from build123d import *

# Parameters (mm, degrees)
SKETCH2_W           = 17
SKETCH2_H           = 21
BOSS_EXTRUDE1_DEPTH = 3
SKETCH4_R           = 1.25
CUT_EXTRUDE1_DEPTH  = 6
SKETCH5_R           = 1.25
CUT_EXTRUDE2_DEPTH  = 6
SKETCH6_W           = 12
SKETCH6_H           = 10
BOSS_EXTRUDE3_DEPTH = 8
SKETCH7_W           = 5
SKETCH7_H           = 4
BOSS_EXTRUDE4_DEPTH = 4
BOSS_EXTRUDE5_DEPTH = 4
SKETCH9_R           = 1
CUT_EXTRUDE3_DEPTH  = 6


with BuildPart() as part:
    # Sketch2 → Boss-Extrude1 (new body)
    with BuildSketch(Plane(origin=(0, 0, 0), x_dir=(1, 0, 0), z_dir=(0, 1, 0))):
        with Locations((8.5, 10.5)):
            Rectangle(SKETCH2_W, SKETCH2_H)
    extrude(amount=BOSS_EXTRUDE1_DEPTH)

    # Sketch4 → Cut-Extrude1 (cut)
    with BuildSketch(Plane(origin=(0, 3, 0), x_dir=(1, 0, 0), z_dir=(0, 1, 0))):
        with Locations(Location((8, 18, 0), (0, 0, 270))):
            Circle(SKETCH4_R)
    extrude(amount=-CUT_EXTRUDE1_DEPTH, mode=Mode.SUBTRACT)

    # Sketch5 → Cut-Extrude2 (cut)
    with BuildSketch(Plane(origin=(0, 3, 0), x_dir=(1, 0, 0), z_dir=(0, 1, 0))):
        with Locations(Location((8, 3, 0), (0, 0, 270))):
            Circle(SKETCH5_R)
    extrude(amount=-CUT_EXTRUDE2_DEPTH, mode=Mode.SUBTRACT)

    # Sketch6 → Boss-Extrude3 (add)
    with BuildSketch(Plane(origin=(0, 3, 0), x_dir=(1, 0, 0), z_dir=(0, 1, 0))):
        with Locations((6, 10.5)):
            Rectangle(SKETCH6_W, SKETCH6_H)
    extrude(amount=BOSS_EXTRUDE3_DEPTH)

    # Sketch7 → Boss-Extrude4 (add)
    with BuildSketch(Plane(origin=(0, 3, 0), x_dir=(1, 0, 0), z_dir=(0, 1, 0))):
        with Locations((14.5, 10.5)):
            Rectangle(SKETCH7_W, SKETCH7_H)
    extrude(amount=BOSS_EXTRUDE4_DEPTH)

    # Sketch8 → Boss-Extrude5 (add)
    with BuildSketch(Plane(origin=(0, 0, -12.5), x_dir=(-1, 0, 0), z_dir=(0, 0, -1))):
        with BuildLine():
            Line((-17, 7), (-12, 7))
            Line((-12, 7), (-12, 11))
            ThreePointArc((-12, 11), (-15.234221224, 9.91777653), (-17, 7))
        make_face()
    extrude(amount=-BOSS_EXTRUDE5_DEPTH)

    # Sketch9 → Cut-Extrude3 (cut)
    with BuildSketch(Plane.XY.offset(-8.5)):
        with Locations((14.174425002, 8.5)):
            Circle(SKETCH9_R)
    extrude(amount=-CUT_EXTRUDE3_DEPTH, mode=Mode.SUBTRACT)


solid = part.part
For this review, take the finished solid that the model builds, in its own axes (mm). A direction names the side the tool comes from. Give positions to 0.01 mm unless a question says otherwise; leave off trailing zeros. Write each loop counter-clockwise with the first axis right and the second up, starting at its lowest first coordinate (ties: lowest second). Pieces come first, ordered by that corner, then holes. Notation, with made-up numbers: (-32, 50.25) -> (-11, 50.25) arc R31 ccw to (-11, 82.25) -> close; hole circle Ø1 at (-2, 4.25). An arc over 180 degrees is marked (long way). Use CSV: the item, a comma, the result in double quotes.
Q1. Tool access review of faces 1 (the face through (6, 7, -5.5)), 2 (the face through (15, 6, -12.5)), 3 (the face through (6, 7, -15.5)): name each direction out of +Z, -Z, +X, -X, +Y, -Y from which nothing blocks a thin tool from reaching the whole face with its end or side.
Conclusion:
face 1,"+Z, +X, -X, +Y"
face 2,"-Z, +X, +Y"
face 3,"-Z, +X, -X, +Y"
Q2. For P1, Ø2.5, axis at x = 14.5, y = 9, coming from the -Z side; P2, Ø2.5, axis at x = 3.5, y = 5, coming from the -Z side; P3, Ø7, axis at x = 11.5, z = -15.5, coming from the +Y side; P4, Ø2.5, axis at x = 5, y = 6.5, coming from the +Z side, all flat-tipped, find the tip position at first contact; note any pin that passes through.
Conclusion:
P1,"z = -12.5"
P2,"z = -15.5"
P3,"y = 11"
P4,"z = -5.5"
Q3. Take a section at C-C, the plane x = 14.25. Write out the cut boundary in (y, z), then the cut area to 3 significant figures.
Conclusion:
outline,"(0, -21) -> (3, -21) -> (3, -12.5) -> (7.5, -12.5) -> (7.5, -8.5) -> (3, -8.5) -> (3, 0) -> (0, 0) -> close; (9.5, -12.5) -> (10.53, -12.5) -> (10.53, -8.5) -> (9.5, -8.5) -> close"
area,"85.1 mm2"
Q4. Take a section at D-D, the plane y = 8. Write out the cut boundary in (x, z).
Conclusion:
outline,"(0, -15.5) -> (12, -15.5) -> (12, -12.5) -> (13.31, -12.5) -> (13.31, -8.5) -> (12, -8.5) -> (12, -5.5) -> (0, -5.5) -> close; (15.04, -12.5) -> (16.69, -12.5) -> (16.69, -8.5) -> (15.04, -8.5) -> close"
Q5. Take a section at A-A, the plane z = -3. Write out the cut boundary in (x, y), then the cut area to 3 significant figures.
Conclusion:
outline,"(0, 0) -> (6.75, 0) -> (6.75, 3) -> (0, 3) -> close; (9.25, 0) -> (17, 0) -> (17, 3) -> (9.25, 3) -> close"
area,"43.5 mm2"
Q6. Mouldability with a two-part tool opening along Z and no side actions: class faces 4 (the face through (15, 6, -8.5)), 5 (the face through (7.521, 1.521, -16.845)), 6 (the face through (0, 4, -10)) as pulls with the +Z half, pulls with the -Z half, needs draft (parallel to the pull), parting line crosses it, or undercut.
Conclusion:
face 4,"pulls with the +Z half"
face 5,"undercut"
face 6,"needs draft"
Q7. To check wall thickness, follow probe 1 along X at (y, z) = (0.7, -18); probe 2 along X at (y, z) = (7.5, -13.5); probe 3 along Y at (x, z) = (11.5, -19). State the ranges of each line that lie inside material, in increasing order. Write a range as [from, to].
Conclusion:
probe 1,"[0, 6.75], [9.25, 17]"
probe 2,"[0, 12]"
probe 3,"[0, 3]"
Q8. Take a section at B-B, the plane y = 5. Write out the cut boundary in (x, z).
Conclusion:
outline,"(0, -15.5) -> (12, -15.5) -> (12, -12.5) -> (17, -12.5) -> (17, -8.5) -> (12, -8.5) -> (12, -5.5) -> (0, -5.5) -> close"
